```python
from build123d import *

# Parameters (mm, degrees)
F0_R      = 28.641111
F1_DEPTH  = 76.2
F2_R      = 22.86
F1_FACE_R = 5.781111
F3_DEPTH  = 152.4


with BuildPart() as f1:
    # F0 (on Front) → F1 (new body)
    with BuildSketch(Plane.XZ):
        Circle(F0_R)
    extrude(amount=F1_DEPTH)

    # F2
    f2_edges = [f1.edges().sort_by_distance(p)[0] for p in [
        (-28.641111, -76.2, 0),
        (28.641111, -38.1, 0),
        (-28.641111, 0, 0),
    ]]
    fillet(f2_edges, radius=F2_R)

    # F1_face (on face) → F3 (join)
    with BuildSketch(Plane(origin=(0, 0, 0), x_dir=(1, 0, 0), z_dir=(0, 1, 0))):
        Circle(F1_FACE_R)
    extrude(amount=-F3_DEPTH)


solid = f1.part
```
Check sheet for the modelled part. Datum: model origin and axes. Units: mm. A direction names the side the tool comes from. Give positions to 0.01 mm unless a question says otherwise; leave off trailing zeros. Write each loop counter-clockwise with the first axis right and the second up, starting at its lowest first coordinate (ties: lowest second). Pieces come first, ordered by that corner, then holes. Notation, with made-up numbers: (61.5, 8.5) - (85.5, 8.5) arc R24 ccw to (85.5, 33.5) - close; hole circle Ø8 at (-38, -19). An arc over 180 degrees is marked (long way). Answer as a JSON object with one key per item and string values. Group by question number.
1) Depth check by flat-ended pin: P1, Ø5, axis at y = -19.5, z = -10.5, coming from the -X side; P2, Ø3, axis at x = 15.5, z = -3.5, coming from the +Y side; P3, Ø2, axis at x = 9, z = -10.5, coming from the -Y side. Enter the tip coordinate at first touch or a pass-through.
2) Sectioned sample at B-B (y = -29.5). Record the cut outline in (x, z).
3) Access from +Z, -Z, +X, -X, +Y, -Y to the whole of each face (thin tool, end or side, straight path). Record for faces 1 (the face through (27.32, -37.89, 8.6)), 2 (the face through (2.668, -113.767, 5.129)).
4) Thickness scan on probe 1 along Z at (x, y) = (0, -46); probe 2 along Y at (x, z) = (-5, 4); probe 3 along Y at (x, z) = (1, 20.5). Record the ranges inside material, lowest first. Write a range as from..to.
5) Sectioned sample at A-A (y = -112.5). Record the cut outline in (x, z), then the cut area to 3 significant figures.
Geometry results:
{
 "1": {"P1": "stops at x = -27.31", "P2": "stops at y = -1.68", "P3": "stops at y = -75.09"},
 "2": {"outline": "circle Ø57.28 at (0, 0)"},
 "3": {"face 1": "+Y, -Y", "face 2": "-Y"},
 "4": {"probe 1": "z = -28.64..28.64", "probe 2": "y = -76.19..-0.01", "probe 3": "y = -70.81..-5.39"},
 "5": {"outline": "circle Ø11.56 at (0, 0)", "area": "105 mm^2"}
}
